Verification items for the finished model (mm, model axes). Coordinates: 2 decimals unless noted, no trailing zeros. Order: outer loops, then holes, each group sorted by start corner. A loop starts at its lowest first (then second) coordinate and runs counter-clockwise, first axis right, second up. Notation, with made-up numbers: (74.25, 27.25) -> (111.25, 27.25) arc R14 cw to (111.25, 36.25) -> close; hole circle Ø8 at (69.25, -1.5). An arc over 180 degrees is marked (long way). Write each question's results on one line, items separated by ' | '. Start each with the question number.
(1) Cross-section at B-B on z = -63.5. Enter the section's corners in (x, y), and give its area (3 significant figures).
(2) Cross-section at A-A on x = 5. Enter the section's corners in (y, z), and give its area (3 significant figures).
(3) Cross-section at C-C on y = 6.5. Give the number of separate pieces and of enclosed holes in the cut face, and give its area (3 significant figures).
(4) Thickness scan on probe 1 along Z at (x, y) = (99.5, 8.5); probe 2 along X at (y, z) = (6.25, -53.5). Record the ranges inside material, lowest first. Write a range as [from, to].
```python
from build123d import *

# Parameters (mm, degrees)
SKETCH2_W                    = 205
SKETCH2_H                    = 205
BOSS_EXTRUDE1_DEPTH          = 20
SKETCH3_W                    = 57
SKETCH3_H                    = 57
CUT_EXTRUDE1_DEPTH           = 147.330106267
LPATTERN1_COUNT              = 3
LPATTERN1_PITCH              = 66
LPATTERN1_COUNT_DIR2         = 3
LPATTERN1_PITCH_DIR2         = 66
CHAMFER1_SIZE                = 2.5
CHAMFER1_SIZE2               = 9.330127019
M3_CLEARANCE_HOLE1_OUTLINE_R = 1.8
M3_CLEARANCE_HOLE1_DEPTH     = 20


# Read off the part's stored shape, not the designer's step: M3 Clearance Hole1
with BuildPart() as part:
    # Sketch2 → Boss-Extrude1 (new body)
    with BuildSketch(Plane(origin=(0, 0, 0), x_dir=(1, 0, 0), z_dir=(0, 1, 0))):
        Rectangle(SKETCH2_W, SKETCH2_H)
    extrude(amount=BOSS_EXTRUDE1_DEPTH)

    # Sketch3 → Cut-Extrude1 (cut, through all)
    with BuildSketch(Plane(origin=(0, 20, 0), x_dir=(1, 0, 0), z_dir=(0, 1, 0))):
        with Locations((-66, 66)):
            Rectangle(SKETCH3_W, SKETCH3_H)
    cut_extrude1 = extrude(amount=-CUT_EXTRUDE1_DEPTH, mode=Mode.SUBTRACT)

    # LPattern1: Cut-Extrude1 3 × 3
    with Locations(*[(i * LPATTERN1_PITCH, 0, j * LPATTERN1_PITCH_DIR2) for i in range(LPATTERN1_COUNT) for j in range(LPATTERN1_COUNT_DIR2) if (i, j) != (0, 0)]):
        add(cut_extrude1, mode=Mode.SUBTRACT)

    # Chamfer1
    chamfer1_edges = [part.edges().sort_by_distance(p)[0] for p in [
        (94.5, 20, 66),
        (66, 20, 94.5),
        (37.5, 20, 66),
        (66, 20, 37.5),
        (-37.5, 20, -66),
        (-66, 20, -94.5),
        (-94.5, 20, -66),
        (-66, 20, -37.5),
        (28.5, 20, -66),
        (0, 20, -94.5),
        (-28.5, 20, -66),
        (0, 20, -37.5),
        (94.5, 20, -66),
        (66, 20, -37.5),
        (37.5, 20, -66),
        (66, 20, -94.5),
        (-37.5, 20, 0),
        (-66, 20, 28.5),
        (-94.5, 20, 0),
        (-66, 20, -28.5),
        (28.5, 20, 0),
        (0, 20, 28.5),
        (-28.5, 20, 0),
        (0, 20, -28.5),
        (94.5, 20, 0),
        (66, 20, 28.5),
        (37.5, 20, 0),
        (66, 20, -28.5),
        (-37.5, 20, 66),
        (-66, 20, 94.5),
        (-94.5, 20, 66),
        (-66, 20, 37.5),
        (28.5, 20, 66),
        (0, 20, 94.5),
        (-28.5, 20, 66),
        (0, 20, 37.5),
    ]]
    chamfer1_side = [part.faces().sort_by_distance(p)[0] for p in [
        (0, 20, 99.600862197),
    ]]
    chamfer(chamfer1_edges, length=CHAMFER1_SIZE, length2=CHAMFER1_SIZE2, reference=chamfer1_side[0])

    # M3 Clearance Hole1 outline → M3 Clearance Hole1 (cut)
    with BuildSketch(Plane(origin=(0, 0, 0), x_dir=(1, 0, 0), z_dir=(0, 1, 0))):
        with Locations((-99.5, -99.5)):
            Circle(M3_CLEARANCE_HOLE1_OUTLINE_R)
        with Locations((99.5, 99.5)):
            Circle(M3_CLEARANCE_HOLE1_OUTLINE_R)
        with Locations((99.5, -99.5)):
            Circle(M3_CLEARANCE_HOLE1_OUTLINE_R)
        with Locations((-99.5, 99.5)):
            Circle(M3_CLEARANCE_HOLE1_OUTLINE_R)
    extrude(amount=M3_CLEARANCE_HOLE1_DEPTH, mode=Mode.SUBTRACT)


solid = part.part
```
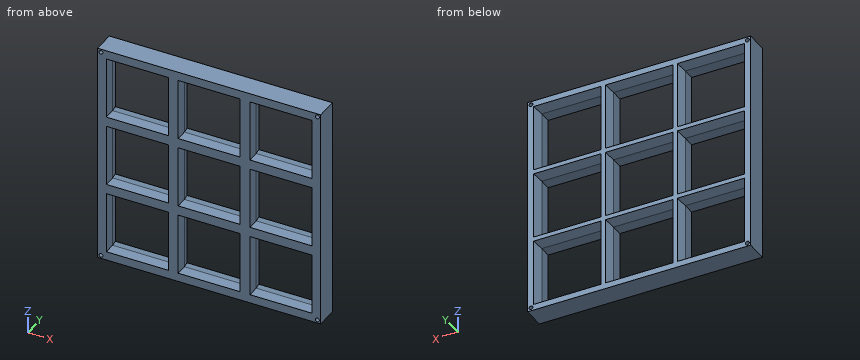
Results are:
1) outline: (-102.5, 0) -> (-94.5, 0) -> (-94.5, 10.67) -> (-97, 20) -> (-102.5, 20) -> close; (-37.5, 0) -> (-28.5, 0) -> (-28.5, 10.67) -> (-31, 20) -> (-35, 20) -> (-37.5, 10.67) -> close; (28.5, 0) -> (37.5, 0) -> (37.5, 10.67) -> (35, 20) -> (31, 20) -> (28.5, 10.67) -> close; (94.5, 0) -> (102.5, 0) -> (102.5, 20) -> (97, 20) -> (94.5, 10.67) -> close | area: 610 mm2
2) outline: (0, -102.5) -> (20, -102.5) -> (20, -97) -> (10.67, -94.5) -> (0, -94.5) -> close; (0, -37.5) -> (10.67, -37.5) -> (20, -35) -> (20, -31) -> (10.67, -28.5) -> (0, -28.5) -> close; (0, 28.5) -> (10.67, 28.5) -> (20, 31) -> (20, 35) -> (10.67, 37.5) -> (0, 37.5) -> close; (0, 94.5) -> (10.67, 94.5) -> (20, 97) -> (20, 102.5) -> (0, 102.5) -> close | area: 610 mm2
3) separate pieces: 1 | enclosed holes: 13 | area: 12,700 mm2
4) probe 1: z = [-102.5, -101.3], [-97.7, 97.7], [101.3, 102.5] | probe 2: x = [-102.5, -94.5], [-37.5, -28.5], [28.5, 37.5], [94.5, 102.5]
